from build123d import *

# Parameters (mm, degrees)
SKETCH_1_R      = 2.1
EXTRUDE_1_DEPTH = 235
FILLET_1_R      = 0.1
FILLET_2_R      = 0.2


with BuildPart() as part:
    # 草图1 → 凸台-拉伸1 (new body)
    with BuildSketch(Plane.XY):
        with BuildLine():
            Line((8.5, -3.9), (-8.5, -3.9))
            ThreePointArc((-8.5, -3.9), (-9.560660172, -3.460660172), (-10, -2.4))
            Line((-10, -2.4), (-10, 4.6))
            ThreePointArc((-10, 4.6), (-9.560660172, 5.660660172), (-8.5, 6.1))
            Line((-8.5, 6.1), (-3.5, 6.1))
            Line((-3.5, 6.1), (-3.5, 5.6))
            Line((-3.5, 5.6), (-3.2, 5.6))
            Line((-3.2, 5.6), (-3.2, 4.3))
            Line((-3.2, 4.3), (-5.2, 4.3))
            Line((-5.2, 4.3), (-5.2, 2))
            Line((-5.2, 2), (-3.2, 0))
            Line((-3.2, 0), (3.2, 0))
            Line((3.2, 0), (5.2, 2))
            Line((5.2, 2), (5.2, 4.3))
            Line((5.2, 4.3), (3.2, 4.3))
            Line((3.2, 4.3), (3.2, 5.6))
            Line((3.2, 5.6), (3.5, 5.6))
            Line((3.5, 5.6), (3.5, 6.1))
            Line((3.5, 6.1), (8.5, 6.1))
            ThreePointArc((8.5, 6.1), (9.560660172, 5.660660172), (10, 4.6))
            Line((10, 4.6), (10, -2.4))
            ThreePointArc((10, -2.4), (9.560660172, -3.460660172), (8.5, -3.9))
        make_face()
        with Locations(Location((-7, -0.9, 0), (0, 0, 180))):
            Circle(SKETCH_1_R, mode=Mode.SUBTRACT)
        with Locations(Location((7, -0.9, 0), (0, 0, 180))):
            Circle(SKETCH_1_R, mode=Mode.SUBTRACT)
    extrude(amount=EXTRUDE_1_DEPTH)

    # 圆角1
    fillet_1_edges = [part.edges().sort_by_distance(p)[0] for p in [
        (3.2, 5.6, 117.5),
        (3.5, 6.1, 117.5),
        (-3.5, 6.1, 117.5),
        (-3.2, 5.6, 117.5),
    ]]
    fillet(fillet_1_edges, radius=FILLET_1_R)

    # 圆角2
    fillet_2_edges = [part.edges().sort_by_distance(p)[0] for p in [
        (5.2, 4.3, 117.5),
        (3.2, 4.3, 117.5),
        (-3.2, 4.3, 117.5),
        (-5.2, 4.3, 117.5),
    ]]
    fillet(fillet_2_edges, radius=FILLET_2_R)


solid = part.part
The model under review builds one solid part; all positions refer to its coordinate system, in mm. Give positions to 0.01 mm unless a question says otherwise; leave off trailing zeros. Write each loop counter-clockwise with the first axis right and the second up, starting at its lowest first coordinate (ties: lowest second). Pieces come first, ordered by that corner, then holes.
1. Draft analysis for pull direction X (two halves, no side actions). For faces 1 (the flat face through (0, -1, 0)), 2 (the flat face through (10, 1, 116)), 3 (the flat face through (0, 0, 116)), state which applies: +X half, -X half, draft (parallel to the pull), parting line (faces both ways), or undercut.
2. Add section A-A, the plane z = 16. Count the separate pieces of the cut face and the enclosed holes in it, plus the area to 3 significant figures.
3. Wall thickness on L1, parallel to X at y = -0.75, z = 154.5; L2, parallel to X at y = 4, z = 178; L3, parallel to Y at x = 7, z = 141.5: over which ranges is each line inside the solid? List them lowest first.
4. Add section B-B, the plane x = 0. Write out the cut boundary in (y, z).
Worked answers:
1. face 1: draft
1. face 2: +X half
1. face 3: undercut
2. separate pieces: 1
2. enclosed holes: 2
2. area: 118 mm2
3. L1: x = -10 to -9.09, -4.91 to 4.91, 9.09 to 10
3. L2: x = -10 to -5.2, 5.2 to 10
3. L3: y = -3.9 to -3, 1.2 to 6.1
4. outline: (-3.9, 0) - (0, 0) - (0, 235) - (-3.9, 235) - close
